```python
from build123d import *

# Parameters (mm, degrees)
SKETCH037_R     = 1.6
SKETCH037_R_2   = 5.65
PAD014_DEPTH    = 2
SKETCH038_R     = 4.1
SKETCH038_R_2   = 1.6
PAD015_DEPTH    = 10
SKETCH039_R     = 1.65
POCKET013_DEPTH = 22.501


with BuildPart() as part:
    # Sketch037 → Pad014 (new body)
    with BuildSketch(Plane.XY):
        with BuildLine():
            ThreePointArc((-16, 13.5), (-12.464466, 14.964466), (-11, 18.5))
            Line((-11, 18.5), (11, 18.5))
            ThreePointArc((11, 18.5), (12.464466, 14.964466), (16, 13.5))
            Line((16, -13.5), (16, 13.5))
            ThreePointArc((16, -13.5), (12.464466, -14.964466), (11, -18.5))
            Line((11, -22.5), (11, -18.5))
            Line((-11, -22.5), (11, -22.5))
            Line((-11, -18.5), (-11, -22.5))
            ThreePointArc((-11, -18.5), (-12.464466, -14.964466), (-16, -13.5))
            Line((-16, 13.5), (-16, -13.5))
        make_face()
        with Locations((-10, 10.5)):
            Circle(SKETCH037_R, mode=Mode.SUBTRACT)
        with Locations((10, 10.5)):
            Circle(SKETCH037_R, mode=Mode.SUBTRACT)
        with Locations((0, -9.5)):
            Circle(SKETCH037_R_2, mode=Mode.SUBTRACT)
        with Locations((0, -19)):
            Circle(SKETCH037_R, mode=Mode.SUBTRACT)
    extrude(amount=-PAD014_DEPTH)

    # Sketch038 → Pad015 (join)
    with BuildSketch(Plane.XY):
        with Locations((-10, 10.5)):
            Circle(SKETCH038_R)
        with Locations((-10, 10.5)):
            Circle(SKETCH038_R_2, mode=Mode.SUBTRACT)
        with Locations((10, 10.5)):
            Circle(SKETCH038_R)
        with Locations((10, 10.5)):
            Circle(SKETCH038_R_2, mode=Mode.SUBTRACT)
        with BuildLine():
            ThreePointArc((-5.05198, -10.5), (0, -14.65), (5.05198, -10.5))
            Line((5.05198, -10.5), (11, -10.5))
            Line((11, -10.5), (11, -22.5))
            Line((11, -22.5), (-11, -22.5))
            Line((-11, -22.5), (-11, -10.5))
            Line((-11, -10.5), (-5.05198, -10.5))
        make_face()
        with Locations((0, -19)):
            Circle(SKETCH038_R_2, mode=Mode.SUBTRACT)
    extrude(amount=PAD015_DEPTH)

    # Sketch039 → Pocket013 (cut, through all)
    with BuildSketch(Plane.XZ):
        with Locations((-8.02599, 5)):
            Circle(SKETCH039_R)
        with Locations((8.02599, 5)):
            Circle(SKETCH039_R)
    extrude(amount=POCKET013_DEPTH, mode=Mode.SUBTRACT)


solid = part.part
```
Build history of the part. All positions in model axes, mm. A direction names the side the tool comes from. Coordinates: 2 decimals unless noted, no trailing zeros. Write each loop counter-clockwise with the first axis right and the second up, starting at its lowest first coordinate (ties: lowest second). Pieces come first, ordered by that corner, then holes.
1. 3-axis set-ups, long thin cutter, end or side, ignore diameter. For faces 1 (the flat face through (-11, -17, 5)), 2 (the cylindrical face through (-0.74, -3.9, -0.99)), 3 (the flat face through (6.66, -10.5, 3.82)): which of +Z, -Z, +X, -X, +Y, -Y reach the whole face in a straight line?
Answer block:
face 1: +Z, -X, -Y
face 2: -Z
face 3: +Z, +X, -X
2. Drill centre lines: probe 1 along Y at (x, z) = (-10, 1); probe 2 along Y at (x, z) = (0, -1.25); probe 3 along Y at (x, z) = (10, -1.55). Where is each one in solid material? Low to high.
Answer block:
probe 1: y = -22.5 to -10.5, 6.4 to 8.9, 12.1 to 14.6
probe 2: y = -22.5 to -20.6, -17.4 to -15.15, -3.85 to 18.5
probe 3: y = -22.5 to 8.9, 12.1 to 18.5
3. Pull direction X, two halves, no side cores. Call faces 4 (the flat face through (16, 0, -1)), 5 (the cylindrical face through (-14.096, 10.68, 4.93)), 6 (the flat face through (0, -16, 10)): released by +X, released by -X, zero draft, split by the parting line, or undercut.
Answer block:
face 4: released by +X
face 5: undercut
face 6: zero draft
4. Band-saw the part on D-D, the plane x = 0. Give the cut face in (y, z).
Answer block:
outline: (-22.5, -2) - (-20.6, -2) - (-20.6, 10) - (-22.5, 10) - close; (-17.4, -2) - (-15.15, -2) - (-15.15, 0) - (-14.65, 0) - (-14.65, 10) - (-17.4, 10) - close; (-3.85, -2) - (18.5, -2) - (18.5, 0) - (-3.85, 0) - close
5. Band-saw the part on C-C, the plane y = -9.5. Give the cut face in (x, z), and give its area (3 significant figures).
Answer block:
outline: (-16, -2) - (-5.65, -2) - (-5.65, 0) - (-16, 0) - close; (5.65, -2) - (16, -2) - (16, 0) - (5.65, 0) - close
area: 41.4 mm2
6. Drop flat-ended pins along their axis: pin 1 (1.8 mm diameter, centred on x = -7.5, z = 4, fed in from +Y); pin 2 (6.5 mm diameter, centred on x = 7.5, z = 5, fed in from +Y); pin 3 (2.5 mm diameter, centred on x = 0.5, y = -13.5, fed in from -Z). Give the stop position or say it passes through.
Answer block:
pin 1: stops at y = 14.27
pin 2: stops at y = 14.6
pin 3: stops at z = 0
7. Band-saw the part on A-A, the plane z = 8. Give the cut face in (x, y).
Answer block:
outline: circle Ø8.2 at (-10, 10.5); (-11, -22.5) - (11, -22.5) - (11, -10.5) - (5.05, -10.5) arc R5.15 cw to (-5.05, -10.5) - (-11, -10.5) - close; circle Ø8.2 at (10, 10.5); hole circle Ø3.2 at (-10, 10.5); hole circle Ø3.2 at (0, -19); hole circle Ø3.2 at (10, 10.5)
8. Band-saw the part on B-B, the plane y = 10.5. Give the cut face in (x, z).
Answer block:
outline: (-16, -2) - (-11.6, -2) - (-11.6, 10) - (-14.1, 10) - (-14.1, 0) - (-16, 0) - close; (-8.4, -2) - (8.4, -2) - (8.4, 10) - (5.9, 10) - (5.9, 0) - (-5.9, 0) - (-5.9, 10) - (-8.4, 10) - close; (11.6, -2) - (16, -2) - (16, 0) - (14.1, 0) - (14.1, 10) - (11.6, 10) - close
